Part model, mm, in its own coordinate system. Face numbers are marked on the shaded views. A direction names the side the tool comes from. Round coordinates to 2 decimals unless told otherwise and drop trailing zeros. Write each loop counter-clockwise with the first axis right and the second up, starting at its lowest first coordinate (ties: lowest second). Pieces come first, ordered by that corner, then holes.
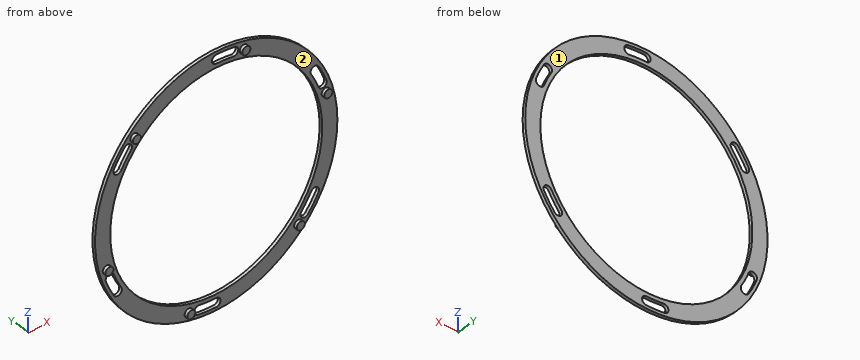
from build123d import *

# Parameters (mm, degrees)
SKETCH1_R           = 200
SKETCH1_R_2         = 175
BOSS_EXTRUDE1_DEPTH = 5
SKETCH2_R           = 2
CUT_EXTRUDE1_DEPTH  = 21
CIRPATTERN1_COUNT   = 6
SCALE1_SCALE        = 0.225
SKETCH3_R           = 1.5
BOSS_EXTRUDE2_DEPTH = 2.26


with BuildPart() as part:
    # Sketch1 → Boss-Extrude1 (new body)
    with BuildSketch(Plane(origin=(0, 0, 0), x_dir=(1, 0, 0), z_dir=(0, 1, 0))):
        Circle(SKETCH1_R)
        Circle(SKETCH1_R_2, mode=Mode.SUBTRACT)
    extrude(amount=BOSS_EXTRUDE1_DEPTH)

    # Sketch2 → Cut-Extrude1 (cut)
    with BuildSketch(Plane(origin=(0, 5, 0), x_dir=(1, 0, 0), z_dir=(0, 1, 0))):
        with Locations((-45.481316373, 182.41559654)):
            Circle(SKETCH2_R)
        with BuildLine():
            ThreePointArc((0, 195), (-15.299523667, 194.398880078), (-30.504720683, 192.599226416))
            ThreePointArc((-30.504720683, 192.599226416), (-36.323497812, 184.590366777), (-28.314638172, 178.771589648))
            ThreePointArc((-28.314638172, 178.771589648), (-14.201096327, 180.442037406), (0, 181))
            ThreePointArc((0, 181), (7, 188), (0, 195))
        make_face()
    cut_extrude1 = extrude(amount=-CUT_EXTRUDE1_DEPTH, mode=Mode.SUBTRACT)

    # CirPattern1: Cut-Extrude1 ×6 about axis
    cirpattern1_axis = Axis((0, 0, 0), (0, 1, 0))
    for i in range(1, CIRPATTERN1_COUNT):
        add(cut_extrude1.rotate(cirpattern1_axis, i * 360 / CIRPATTERN1_COUNT), mode=Mode.SUBTRACT)


with BuildPart() as part_1:
    # Scale1: scaled about (0, 2.5, 0)
    add(part.part.scale(SCALE1_SCALE).moved(Location((0, 1.9375, 0))))

    # Sketch3 → Boss-Extrude2 (add)
    with BuildSketch(Plane(origin=(0, 3.0625, 0), x_dir=(1, 0, 0), z_dir=(0, 1, 0))):
        with Locations((-10.233296184, 41.043509221)):
            Circle(SKETCH3_R)
        with Locations((30.428073554, 29.38404907)):
            Circle(SKETCH3_R)
        with Locations((40.661369738, -11.659460151)):
            Circle(SKETCH3_R)
        with Locations((10.233296184, -41.043509221)):
            Circle(SKETCH3_R)
        with Locations((-30.428073554, -29.38404907)):
            Circle(SKETCH3_R)
        with Locations((-40.661369738, 11.659460151)):
            Circle(SKETCH3_R)
    extrude(amount=-BOSS_EXTRUDE2_DEPTH)


solid = part_1.part
Q1. Tool access for the marked faces 1 and 2: list every direction of +Z, -Z, +X, -X, +Y, -Y with a clear straight run to the whole face (end or side of a thin tool).
Q2. Wall check: line 1 (Z direction, x = 0, y = 2.6) (3 decimals); line 2 (X direction, y = 2.15, z = -1); line 3 (X direction, y = 2.3, z = 22). Give the ranges that are in metal, low to high.
Q3. Saw through at B-B, the plane y = 2.7. Give the number of separate pieces and of enclosed holes in the cut face, and give its area (3 significant figures).
Q4. Saw through at C-C, the plane x = 17. Write the cut outline in (y, z).
Q5. Saw through at A-A, the plane z = -8. Write the cut outline in (x, y).
Computed:
1. face 1: +Z, -Z, +X, -X, +Y
1. face 2: -Y
2. line 1: z = -45 to -43.875, -40.725 to -39.375, 39.375 to 40.725, 43.875 to 45
2. line 2: x = -44.99 to -39.36, 39.36 to 44.99
2. line 3: x = -39.26 to -37.96, -34.27 to -32.66, 32.66 to 35.31, 37.96 to 39.26
3. separate pieces: 1
3. enclosed holes: 7
3. area: 1,320 mm2
4. outline: (1.94, -41.67) - (3.06, -41.67) - (3.06, -35.52) - (1.94, -35.52) - close; (1.94, 35.52) - (3.06, 35.52) - (3.06, 41.67) - (1.94, 41.67) - close
5. outline: (-44.28, 1.94) - (-38.55, 1.94) - (-38.55, 3.06) - (-44.28, 3.06) - close; (38.55, 1.94) - (44.28, 1.94) - (44.28, 3.06) - (38.55, 3.06) - close
